Model file for the job. Use its own axes, mm. Face numbers are marked on the shaded views. A direction names the side the tool comes from. Round coordinates to 2 decimals unless told otherwise and drop trailing zeros. Order: outer loops, then holes, each group sorted by start corner. A loop starts at its lowest first (then second) coordinate and runs counter-clockwise, first axis right, second up. Notation, with made-up numbers: (-28.75, 43.25) - (-19.75, 43.25) arc R18 cw to (-19.75, 52.25) - close; hole circle Ø11 at (78, -29.5). An arc over 180 degrees is marked (long way). Put each result on its own line as item: value. Start each with the question number.
Item 1: Saw through at A-A on x = 4. List the corners of the cut face in (y, z).
Item 2: Mould opens along Y. For the marked faces 1, 2 and 3 say: pulls with the +Y half, pulls with the -Y half, needs draft (parallel to the pull), parting line crosses it, or undercut.
Item 3: Pin check, flat tips, straight feed: pin 1 Ø3 at (x, y) = (-2.5, 1.5) entering from +Z; pin 2 Ø0.6 at (y, z) = (1, 4) entering from +X; pin 3 Ø0.9 at (y, z) = (-1.5, 4.5) entering from -X; pin 4 Ø1 at (x, z) = (-7.5, 4.5) entering from +Y. Stop position of each tip, or through.
Item 4: Saw through at D-D on z = 1.5. List the corners of the cut face in (x, y).
Item 5: Which spindle directions (+Z, -Z, +X, -X, +Y, -Y) get a long thin tool onto all of the face, cutting with end or side? Do the marked faces 4, 5, 6, 7 and 8. Say none if no direction does.
Item 6: Saw through at B-B on y = -3.5. List the corners of the cut face in (x, z) (3 decimals).
Item 7: Probe probe 1 along X at (y, z) = (1.5, 8.25); probe 2 along X at (y, z) = (-3.25, 8.5) (3 decimals); probe 3 along X at (y, z) = (-1.75, 4.5). List the from-to ranges inside material, lowest first.
Item 8: Saw through at C-C on z = 3. State how many separate pieces and enclosed holes the cut face has, plus the area to 3 significant figures.
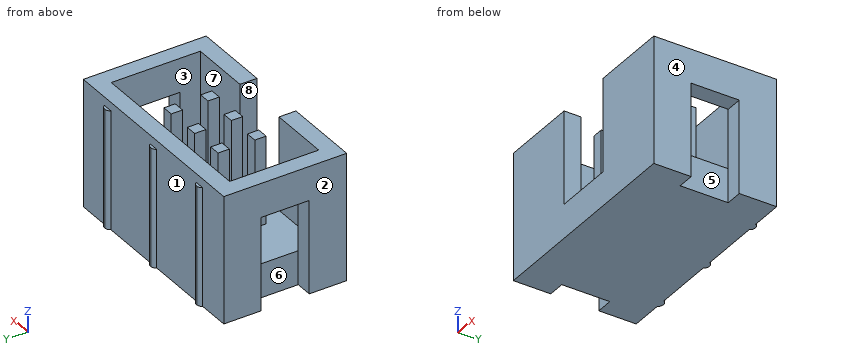
```python
from build123d import *

# Parameters (mm, degrees)
SKICA1_W                 = 15.3
SKICA1_H                 = 8.7
P_IDAT_VYSUNUT_M1_DEPTH  = 9
SKICA2_W                 = 12.9
SKICA2_H                 = 6.3
ODEBRAT_VYSUNUT_M1_DEPTH = 6.6
SKICA3_W                 = 4.25
SKICA3_H                 = 6.6
ODEBRAT_VYSUNUT_M2_DEPTH = 6.6
SKICA4_W                 = 6.6
SKICA4_H                 = 3.4
ODEBRAT_VYSUNUT_M3_DEPTH = 1.2
SKICA5_W                 = 6.6
SKICA5_H                 = 3.4
ODEBRAT_VYSUNUT_M4_DEPTH = 1.2
SKICA6_W                 = 0.7
SKICA6_H                 = 8.4
SKICA6_H_2               = 8.384805524
P_IDAT_VYSUNUT_M2_DEPTH  = 0.2
ZAOBLIT2_R               = 0.35
ZAOBLIT3_R               = 0.35
SKICA7_W                 = 0.8
SKICA7_H                 = 0.8
P_IDAT_VYSUNUT_M3_DEPTH  = 6.2


with BuildPart() as part:
    # Skica1 → Přidat vysunutím1 (new body)
    with BuildSketch(Plane.XY):
        Rectangle(SKICA1_W, SKICA1_H)
    extrude(amount=P_IDAT_VYSUNUT_M1_DEPTH)

    # Skica2 → Odebrat vysunutím1 (cut)
    with BuildSketch(Plane.XY.offset(9)):
        Rectangle(SKICA2_W, SKICA2_H)
    extrude(amount=-ODEBRAT_VYSUNUT_M1_DEPTH, mode=Mode.SUBTRACT)

    # Skica3 → Odebrat vysunutím2 (cut)
    with BuildSketch(Plane(origin=(0, -4.35, 0), x_dir=(-1, 0, 0), z_dir=(0, -1, 0))):
        with Locations((0, -5.7)):
            Rectangle(SKICA3_W, SKICA3_H)
    extrude(amount=-ODEBRAT_VYSUNUT_M2_DEPTH, mode=Mode.SUBTRACT)

    # Skica4 → Odebrat vysunutím3 (cut)
    with BuildSketch(Plane.ZY.offset(7.65)):
        with Locations((3.3, 0)):
            Rectangle(SKICA4_W, SKICA4_H)
    extrude(amount=-ODEBRAT_VYSUNUT_M3_DEPTH, mode=Mode.SUBTRACT)

    # Skica5 → Odebrat vysunutím4 (cut)
    with BuildSketch(Plane(origin=(7.65, 0, 0), x_dir=(0, 0, -1), z_dir=(1, 0, 0))):
        with Locations((-3.3, 0)):
            Rectangle(SKICA5_W, SKICA5_H)
    extrude(amount=-ODEBRAT_VYSUNUT_M4_DEPTH, mode=Mode.SUBTRACT)

    # Skica6 → Přidat vysunutím2 (add)
    with BuildSketch(Plane(origin=(0, 4.35, 0), x_dir=(1, 0, 0), z_dir=(0, 1, 0))):
        with Locations((5, -4.2)):
            Rectangle(SKICA6_W, SKICA6_H)
        with Locations((0, -4.192402762)):
            Rectangle(SKICA6_W, SKICA6_H_2)
        with Locations((-5, -4.192402762)):
            Rectangle(SKICA6_W, SKICA6_H_2)
    extrude(amount=P_IDAT_VYSUNUT_M2_DEPTH)

    # Zaoblit2
    # the kernel refuses this fillet: 0.35 mm, written as the material it takes off along each edge
    with BuildSketch(Plane(origin=(5.35, 4.55, 9.190569415), x_dir=(0, -1, 0), z_dir=(0, 0, -1))) as zaoblit2_piece_1:
        with BuildLine():
            CenterArc((0.35, 0.316227766), ZAOBLIT2_R, 180, 64.623066475)
            Line((0, 0.316227766), (-0.007, 0.316227766))
            Line((-0.007, 0.316227766), (-0.007, 0))
            Line((-0.007, 0), (0, -0.007))
            ThreePointArc((0, -0.007), (0.1, -0.007), (0.197, -0.006324555))
            Line((0.197, -0.006324555), (0.2, 0))
        make_face()
    extrude(amount=9.98113883, mode=Mode.SUBTRACT)

    # Zaoblit3
    # the kernel refuses this fillet: 0.35 mm, written as the material it takes off along each edge
    with BuildSketch(Plane(origin=(-5.35, 4.55, 9.175374939), x_dir=(1, 0, 0), z_dir=(0, 0, -1))) as zaoblit3_piece_1:
        with BuildLine():
            CenterArc((0.316227766, 0.35), ZAOBLIT3_R, 205.376933525, 64.623066475)
            Line((0, 0.2), (-0.006324555, 0.197))
            ThreePointArc((-0.006324555, 0.197), (-0.007, 0.1), (-0.007, 0))
            Line((-0.007, 0), (0, -0.007))
            Line((0, -0.007), (0.316227766, -0.007))
            Line((0.316227766, -0.007), (0.316227766, 0))
        make_face()
    extrude(amount=9.965944354, mode=Mode.SUBTRACT)
    with BuildSketch(Plane(origin=(-4.65, 4.55, -0.790569415), x_dir=(0, -1, 0), z_dir=(0, 0, 1))) as zaoblit3_piece_2:
        with BuildLine():
            CenterArc((0.35, -0.316227766), ZAOBLIT3_R, 115.376933525, 64.623066475)
            Line((0, -0.316227766), (-0.007, -0.316227766))
            Line((-0.007, -0.316227766), (-0.007, 0))
            Line((-0.007, 0), (0, 0.007))
            ThreePointArc((0, 0.007), (0.1, 0.007), (0.197, 0.006324555))
            Line((0.197, 0.006324555), (0.2, 0))
        make_face()
    extrude(amount=9.965944354, mode=Mode.SUBTRACT)
    with BuildSketch(Plane(origin=(-0.35, 4.55, -0.790569415), x_dir=(1, 0, 0), z_dir=(0, 0, 1))) as zaoblit3_piece_3:
        with BuildLine():
            CenterArc((0.316227766, -0.35), ZAOBLIT3_R, 90, 64.623066475)
            Line((0, -0.2), (-0.006324555, -0.197))
            ThreePointArc((-0.006324555, -0.197), (-0.007, -0.1), (-0.007, 0))
            Line((-0.007, 0), (0, 0.007))
            Line((0, 0.007), (0.316227766, 0.007))
            Line((0.316227766, 0.007), (0.316227766, 0))
        make_face()
    extrude(amount=9.965944354, mode=Mode.SUBTRACT)
    with BuildSketch(Plane(origin=(0.35, 4.55, 9.175374939), x_dir=(0, -1, 0), z_dir=(0, 0, -1))) as zaoblit3_piece_4:
        with BuildLine():
            CenterArc((0.35, 0.316227766), ZAOBLIT3_R, 180, 64.623066475)
            Line((0, 0.316227766), (-0.007, 0.316227766))
            Line((-0.007, 0.316227766), (-0.007, 0))
            Line((-0.007, 0), (0, -0.007))
            ThreePointArc((0, -0.007), (0.1, -0.007), (0.197, -0.006324555))
            Line((0.197, -0.006324555), (0.2, 0))
        make_face()
    extrude(amount=9.965944354, mode=Mode.SUBTRACT)
    with BuildSketch(Plane(origin=(4.65, 4.55, -0.790569415), x_dir=(0, -1, 0), z_dir=(0, 0, 1))) as zaoblit3_piece_5:
        with BuildLine():
            CenterArc((0.35, 0.316227766), ZAOBLIT3_R, 180, 64.623066475)
            Line((0, 0.316227766), (-0.007, 0.316227766))
            Line((-0.007, 0.316227766), (-0.007, 0))
            Line((-0.007, 0), (0, -0.007))
            ThreePointArc((0, -0.007), (0.1, -0.007), (0.197, -0.006324555))
            Line((0.197, -0.006324555), (0.2, 0))
        make_face()
    extrude(amount=9.98113883, mode=Mode.SUBTRACT)

    # Skica7 → Přidat vysunutím3 (add)
    with BuildSketch(Plane.XY.offset(2.4)):
        with Locations((-2.55, -1.3)):
            Rectangle(SKICA7_W, SKICA7_H)
        with Locations((-2.55, 1.3)):
            Rectangle(SKICA7_W, SKICA7_H)
        with Locations((0, -1.3)):
            Rectangle(SKICA7_W, SKICA7_H)
        with Locations((2.55, -1.3)):
            Rectangle(SKICA7_W, SKICA7_H)
        with Locations((2.55, 1.3)):
            Rectangle(SKICA7_W, SKICA7_H)
        with Locations((0, 1.3)):
            Rectangle(SKICA7_W, SKICA7_H)
    extrude(amount=P_IDAT_VYSUNUT_M3_DEPTH)


solid = part.part
```
Results found:
1. outline: (-4.35, 0) - (4.35, 0) - (4.35, 9) - (3.15, 9) - (3.15, 2.4) - (-3.15, 2.4) - (-3.15, 9) - (-4.35, 9) - close
2. face 1: pulls with the +Y half
2. face 2: needs draft
2. face 3: undercut
3. pin 1: stops at z = 8.6
3. pin 2: stops at x = 2.95
3. pin 3: stops at x = -7.65
3. pin 4: stops at y = 4.35
4. outline: (-7.65, -4.35) - (7.65, -4.35) - (7.65, -1.7) - (6.45, -1.7) - (6.45, 1.7) - (7.65, 1.7) - (7.65, 4.35) - (5.35, 4.35) arc R0.35 ccw to (5.03, 4.55) - (4.97, 4.55) arc R0.35 ccw to (4.65, 4.35) - (0.35, 4.35) arc R0.35 ccw to (0.03, 4.55) - (-0.03, 4.55) arc R0.35 ccw to (-0.35, 4.35) - (-4.65, 4.35) arc R0.35 ccw to (-4.97, 4.55) - (-5.03, 4.55) arc R0.35 ccw to (-5.35, 4.35) - (-7.65, 4.35) - (-7.65, 1.7) - (-6.45, 1.7) - (-6.45, -1.7) - (-7.65, -1.7) - close
5. face 4: +Z, -Z, +X, +Y, -Y
5. face 5: -Z, +X
5. face 6: -Z, -X
5. face 7: +Z
5. face 8: +Z, -Y
6. outline: (-7.65, 0) - (7.65, 0) - (7.65, 9) - (2.125, 9) - (2.125, 2.4) - (-2.125, 2.4) - (-2.125, 9) - (-7.65, 9) - close
7. probe 1: x = -7.65 to -6.45, -2.95 to -2.15, -0.4 to 0.4, 2.15 to 2.95, 6.45 to 7.65
7. probe 2: x = -7.65 to -2.125, 2.125 to 7.65
7. probe 3: x = -7.65 to -6.45, 6.45 to 7.65
8. separate pieces: 9
8. enclosed holes: 0
8. area: 42.7 mm²
